The drawing under review shows one solid part. Ordinate dimensions are in mm from its lowest x, y, z. Round coordinates to 2 decimals unless told otherwise and drop trailing zeros. Order: outer loops, then holes, each group sorted by start corner. A loop starts at its lowest first (then second) coordinate and runs counter-clockwise, first axis right, second up. Notation, with made-up numbers: (3.5, 22.25) - (54.5, 22.25) arc R19 cw to (54.5, 53.25) - close; hole circle Ø6 at (-18, 89). An arc over 180 degrees is marked (long way). Answer as a JSON object with one key per item and string values. Group by question number.
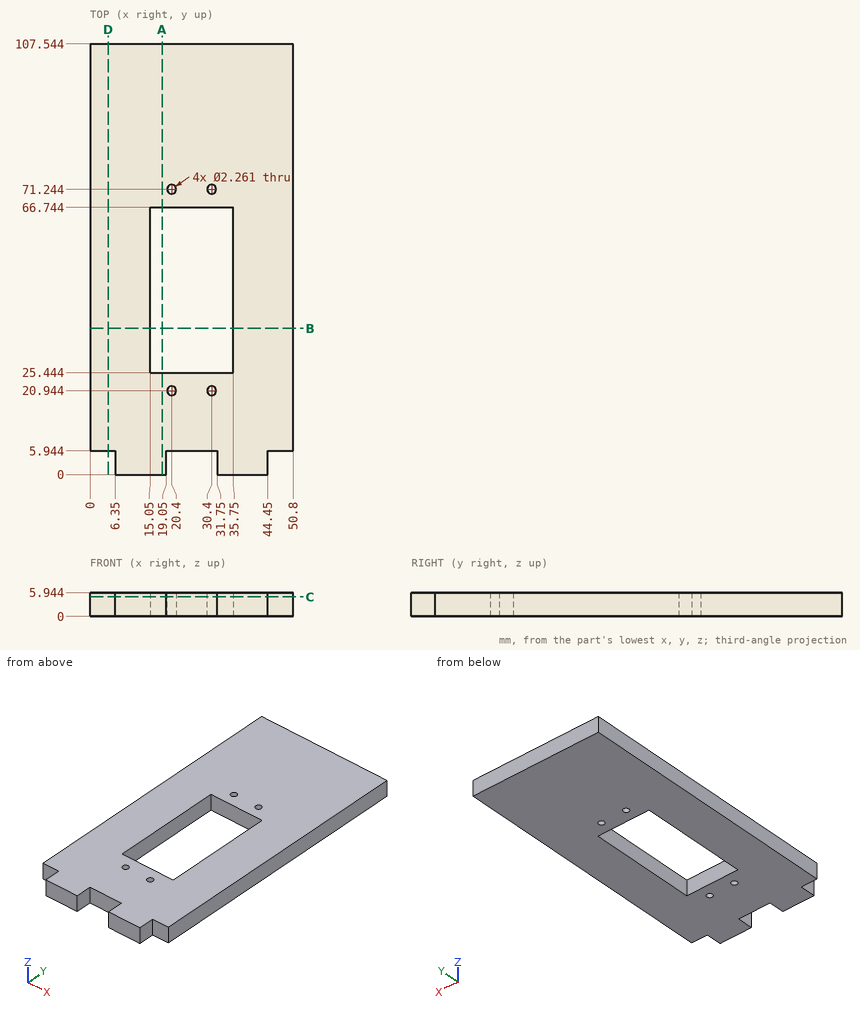
1. Take a section at A-A, the plane x = 18. Give the boundary of the cut face in (y, z), then the cut area to 3 significant figures.
2. Take a section at D-D, the plane x = 4.5. Give the boundary of the cut face in (y, z), then the cut area to 3 significant figures.
3. To check wall thickness, follow line 1 (Y direction, x = 20.4, z = 1.7); line 2 (X direction, y = 63, z = 1.45); line 3 (Y direction, x = 18.5, z = 4.7). State the ranges of each line that lie inside material, in increasing order. Write a range as from..to.
4. Take a section at C-C, the plane z = 4.9. Give the boundary of the cut face in (x, y).
5. Take a section at B-B, the plane y = 36.5. Give the boundary of the cut face in (x, z).
6. Clearance check with flat-ended pins moving along their axes: P1, Ø1.4, axis at x = 30.4, y = 71.24, coming from the +Z side; P2, Ø5, axis at x = 44, y = 44.5, coming from the -Z side; P3, Ø3, axis at y = 2.5, z = 3, coming from the -X side; P4, Ø1.8, axis at x = 49, z = 2.5, coming from the -Y side. State where each tip first meets the part, or that it passes through.
Response values:
{
 "1": {"outline": "(0, 0) - (25.44, 0) - (25.44, 5.94) - (0, 5.94) - close; (66.74, 0) - (107.54, 0) - (107.54, 5.94) - (66.74, 5.94) - close", "area": "394 mm2"},
 "2": {"outline": "(5.94, 0) - (107.54, 0) - (107.54, 5.94) - (5.94, 5.94) - close", "area": "604 mm2"},
 "3": {"line 1": "5.94..19.81, 22.07..25.44, 66.74..70.11, 72.37..107.54", "line 2": "0..15.05, 35.75..50.8", "line 3": "0..25.44, 66.74..107.54"},
 "4": {"outline": "(0, 5.94) - (6.35, 5.94) - (6.35, 0) - (19.05, 0) - (19.05, 5.94) - (31.75, 5.94) - (31.75, 0) - (44.45, 0) - (44.45, 5.94) - (50.8, 5.94) - (50.8, 107.54) - (0, 107.54) - close; hole (15.05, 25.44) - (35.75, 25.44) - (35.75, 66.74) - (15.05, 66.74) - close; hole circle Ø2.26 at (20.4, 20.94); hole circle Ø2.26 at (20.4, 71.24); hole circle Ø2.26 at (30.4, 20.94); hole circle Ø2.26 at (30.4, 71.24)"},
 "5": {"outline": "(0, 0) - (15.05, 0) - (15.05, 5.94) - (0, 5.94) - close; (35.75, 0) - (50.8, 0) - (50.8, 5.94) - (35.75, 5.94) - close"},
 "6": {"P1": "through", "P2": "z = 0", "P3": "x = 6.35", "P4": "y = 5.94"}
}
